```python
from build123d import *

# Parameters (mm, degrees)
BOSS_EXTRUDE1_DEPTH = 6.35
SKETCH2_R           = 1.905
CUT_EXTRUDE1_DEPTH  = 7.35
CUT_EXTRUDE2_REACH  = 18.51
SKETCH3_R           = 1.27


with BuildPart() as part:
    # Sketch1 → Boss-Extrude1 (new body)
    with BuildSketch(Plane.XY):
        Polygon((0, 0), (0, -35.052), (6.35, -35.052), (6.35, -6.35), (16.51, -6.35), (16.51, 0), align=None)
    extrude(amount=BOSS_EXTRUDE1_DEPTH)

    # Sketch2 → Cut-Extrude1 (cut, through all)
    with BuildSketch(Plane.XY.offset(6.35)):
        with Locations((3.175, -31.877)):
            Circle(SKETCH2_R)
    extrude(amount=-CUT_EXTRUDE1_DEPTH, mode=Mode.SUBTRACT)

    # Sketch3 → Cut-Extrude2 (cut, up to next)
    with BuildSketch(Plane.ZY, mode=Mode.PRIVATE) as cut_extrude2_sk1:
        with Locations((3.175, -31.877)):
            Circle(SKETCH3_R)
    cut_extrude2_tool1 = extrude(cut_extrude2_sk1.sketch, amount=-CUT_EXTRUDE2_REACH, mode=Mode.PRIVATE) & part.part
    add(cut_extrude2_tool1.solids().sort_by_distance((0, -31.877, 3.175))[0], mode=Mode.SUBTRACT)


solid = part.part
```
Here's how the part is built. I have some questions about the finished solid (model axes, mm). A direction names the side the tool comes from. Coordinates: 2 decimals unless noted, no trailing zeros. Write each loop counter-clockwise with the first axis right and the second up, starting at its lowest first coordinate (ties: lowest second). Pieces come first, ordered by that corner, then holes. Notation, with made-up numbers: (58.25, 30) - (108.25, 30) arc R20 cw to (108.25, 50) - close; hole circle Ø2 at (4, 71). An arc over 180 degrees is marked (long way). One line per item, written item: value.
1) On a 3-axis mill with a long thin cutter (end or side, diameter ignored), from which of +Z, -Z, +X, -X, +Y, -Y can I reach the whole of each face in a straight line? I mean faces 1 (the flat face through (11, -6.35, 3)), 2 (the flat face through (0, -17, 3)). Say none if no direction works.
Model answer:
face 1: +Z, -Z, +X, -Y
face 2: +Z, -Z, -X, +Y, -Y
2) Suppose I cut it at C-C on x = 9.5. Write out the boundary of the cut face in (y, z).
Model answer:
outline: (-6.35, 0) - (0, 0) - (0, 6.35) - (-6.35, 6.35) - close
3) Suppose I cut it at B-B on z = 3.25. Write out the boundary of the cut face in (x, y) (3 decimals).
Model answer:
outline: (0, -35.052) - (6.35, -35.052) - (6.35, -6.35) - (16.51, -6.35) - (16.51, 0) - (0, 0) - (0, -30.609) - (1.753, -30.609) arc R1.905 cw (long way) to (1.753, -33.145) - (0, -33.145) - close
4) Suppose I cut it at A-A on z = 0.5. Write out the boundary of the cut face in (x, y) (3 decimals).
Model answer:
outline: (0, -35.052) - (6.35, -35.052) - (6.35, -6.35) - (16.51, -6.35) - (16.51, 0) - (0, 0) - close; hole circle Ø3.81 at (3.175, -31.877)
5) I need wall thicknesses on line 1 along X through (y, z) = (-26.5, 6); line 2 along Y through (x, z) = (1.75, 1.5); line 3 along Y through (x, z) = (14.25, 2). Which ranges of each line are inside material? Lowest first, please.
Model answer:
line 1: x = 0 to 6.35
line 2: y = -35.05 to -33.14, -30.61 to 0
line 3: y = -6.35 to 0
6) I'm going to push flat-ended pins straight in: P1, Ø3, axis at y = -21, z = 4, coming from the +X side; P2, Ø1.9, axis at x = 10.5, z = 4.5, coming from the -Y side. Where does each tip first touch, or does it pass through?
Model answer:
P1: stops at x = 6.35
P2: stops at y = -6.35
7) We'd pull the mould along Y, two halves only. Please class faces 3 (the cylindrical face through (0.67, -31.02, 2.24)), 4 (the flat face through (3, -35.052, 3)), 5 (the flat face through (6.35, -21, 3)): pulls with the +Y half, pulls with the -Y half, needs draft (parallel to the pull), parting line crosses it, or undercut.
Model answer:
face 3: undercut
face 4: pulls with the -Y half
face 5: needs draft
8) Suppose I cut it at D-D on y = -15.5. Write out the boundary of the cut face in (x, z), and give its area (3 significant figures).
Model answer:
outline: (0, 0) - (6.35, 0) - (6.35, 6.35) - (0, 6.35) - close
area: 40.3 mm²
